from build123d import *

# Parameters (mm, degrees)
SKETCH1_W           = 457.2
SKETCH1_H           = 304.8
BOSS_EXTRUDE1_DEPTH = 3.175
CUT_EXTRUDE1_DEPTH  = 4.175
CUT_EXTRUDE2_REACH  = 5.175
SKETCH5_R           = 1.700000029
CUT_EXTRUDE3_DEPTH  = 4.175
SKETCH7_R           = 2.200000045
CUT_EXTRUDE5_DEPTH  = 4.175
SKETCH8_R           = 1.000000032
CUT_EXTRUDE6_DEPTH  = 4.175
SKETCH12_R          = 1.700000029
CUT_EXTRUDE7_DEPTH  = 4.175
SKETCH13_R          = 1.700000029
SKETCH13_R_2        = 1.127000032
CUT_EXTRUDE8_DEPTH  = 4.175
SKETCH14_R          = 2.200000045
SKETCH14_R_2        = 1.700000029
SKETCH14_R_3        = 2.499999953
CUT_EXTRUDE9_DEPTH  = 4.175


with BuildPart() as part:
    # Sketch1 → Boss-Extrude1 (new body)
    with BuildSketch(Plane(origin=(0, 0, 0), x_dir=(1, 0, 0), z_dir=(0, 1, 0))):
        Rectangle(SKETCH1_W, SKETCH1_H)
    extrude(amount=BOSS_EXTRUDE1_DEPTH)

    # Sketch2 → Cut-Extrude1 (cut, through all)
    with BuildSketch(Plane(origin=(0, 3.175, 0), x_dir=(1, 0, 0), z_dir=(0, 1, 0))):
        with BuildLine():
            Line((-218.100000045, 66.04), (-218.100000045, 66.675))
            ThreePointArc((-218.100000045, 66.675), (-215.9, 68.875000045), (-213.699999955, 66.675))
            Line((-213.699999955, 66.675), (-213.699999955, 66.04))
            ThreePointArc((-213.699999955, 66.04), (-215.9, 63.839999955), (-218.100000045, 66.04))
        make_face()
        with BuildLine():
            Line((-186.350000045, 66.04), (-186.350000045, 66.675))
            ThreePointArc((-186.350000045, 66.675), (-184.15, 68.875000045), (-181.949999955, 66.675))
            Line((-181.949999955, 66.675), (-181.949999955, 66.04))
            ThreePointArc((-181.949999955, 66.04), (-184.15, 63.839999955), (-186.350000045, 66.04))
        make_face()
        with BuildLine():
            Line((-213.699999955, -66.04), (-213.699999955, -66.675))
            ThreePointArc((-213.699999955, -66.675), (-215.9, -68.875000045), (-218.100000045, -66.675))
            Line((-218.100000045, -66.675), (-218.100000045, -66.04))
            ThreePointArc((-218.100000045, -66.04), (-215.9, -63.839999955), (-213.699999955, -66.04))
        make_face()
        with BuildLine():
            Line((-181.949999955, -66.04), (-181.949999955, -66.675))
            ThreePointArc((-181.949999955, -66.675), (-184.15, -68.875000045), (-186.350000045, -66.675))
            Line((-186.350000045, -66.675), (-186.350000045, -66.04))
            ThreePointArc((-186.350000045, -66.04), (-184.15, -63.839999955), (-181.949999955, -66.04))
        make_face()
    extrude(amount=-CUT_EXTRUDE1_DEPTH, mode=Mode.SUBTRACT)

    # Sketch4 → Cut-Extrude2 (cut, up to next)
    with BuildSketch(Plane(origin=(0, 3.175, 0), x_dir=(1, 0, 0), z_dir=(0, 1, 0)), mode=Mode.PRIVATE) as cut_extrude2_sk1:
        with BuildLine():
            Line((-185.7375, 46.0375), (-185.7375, -46.0375))
            Line((-185.7375, -46.0375), (-180.34, -46.0375))
            ThreePointArc((-180.34, -46.0375), (-179.666480791, -46.316480791), (-179.3875, -46.99))
            Line((-179.3875, -46.99), (-179.3875, -55.3085))
            Line((-179.3875, -55.3085), (-70.0405, -55.3085))
            Line((-70.0405, -55.3085), (-70.0405, 55.3085))
            Line((-70.0405, 55.3085), (-179.3875, 55.3085))
            Line((-179.3875, 55.3085), (-179.3875, 46.99))
            ThreePointArc((-179.3875, 46.99), (-179.666480791, 46.316480791), (-180.34, 46.0375))
            Line((-180.34, 46.0375), (-185.7375, 46.0375))
        make_face()
    cut_extrude2_tool1 = extrude(cut_extrude2_sk1.sketch, amount=-CUT_EXTRUDE2_REACH, mode=Mode.PRIVATE) & part.part
    add(cut_extrude2_tool1.solids().sort_by_distance((-127.382939, 3.175, 0))[0], mode=Mode.SUBTRACT)

    # Sketch5 → Cut-Extrude3 (cut, through all)
    with BuildSketch(Plane(origin=(0, 3.175, 0), x_dir=(1, 0, 0), z_dir=(0, 1, 0))):
        with Locations((-203.2, 79.629)):
            Circle(SKETCH5_R)
        with Locations((-222.25, 143.129)):
            Circle(SKETCH5_R)
        with Locations((-222.25, 79.629)):
            Circle(SKETCH5_R)
        with Locations((-203.2, -79.629)):
            Circle(SKETCH5_R)
        with Locations((-222.25, -79.629)):
            Circle(SKETCH5_R)
        with Locations((-222.25, -143.129)):
            Circle(SKETCH5_R)
    extrude(amount=-CUT_EXTRUDE3_DEPTH, mode=Mode.SUBTRACT)

    # Sketch7 → Cut-Extrude5 (cut, through all)
    with BuildSketch(Plane(origin=(0, 3.175, 0), x_dir=(1, 0, 0), z_dir=(0, 1, 0))):
        with Locations((-50.720000033, -132.250000041)):
            Circle(SKETCH7_R)
        with Locations((-40.719999967, -132.250000041)):
            Circle(SKETCH7_R)
        with Locations((-50.720000033, -83.649999959)):
            Circle(SKETCH7_R)
        with Locations((-40.719999967, -83.649999959)):
            Circle(SKETCH7_R)
        Polygon((-55.846999939, -87.373000006), (-46.22, -87.373000006), (-46.22, -80.769000006), (-45.22, -80.769000006), (-45.22, -87.373000006), (-35.593000061, -87.373000006), (-35.593000061, -128.526999994), (-45.22, -128.526999994), (-45.22, -135.130999994), (-46.22, -135.130999994), (-46.22, -128.526999994), (-55.846999939, -128.526999994), align=None)
    cut_extrude5 = extrude(amount=-CUT_EXTRUDE5_DEPTH, mode=Mode.SUBTRACT)

    # Mirror1: Cut-Extrude5 across plane
    add(cut_extrude5.mirror(Plane.XY), mode=Mode.SUBTRACT)

    # Sketch8 → Cut-Extrude6 (cut, through all)
    with BuildSketch(Plane(origin=(0, 3.175, 0), x_dir=(1, 0, 0), z_dir=(0, 1, 0))):
        with Locations((-63.6905, -38.1)):
            Circle(SKETCH8_R)
        with Locations((-63.6905, -12.7)):
            Circle(SKETCH8_R)
        with Locations((-63.6905, 12.7)):
            Circle(SKETCH8_R)
        with Locations((-63.6905, 38.1)):
            Circle(SKETCH8_R)
    extrude(amount=-CUT_EXTRUDE6_DEPTH, mode=Mode.SUBTRACT)

    # Sketch12 → Cut-Extrude7 (cut, through all)
    with BuildSketch(Plane(origin=(0, 3.175, 0), x_dir=(1, 0, 0), z_dir=(0, 1, 0))):
        with Locations((195.024, -95.25)):
            Circle(SKETCH12_R)
        with Locations((182.324, -95.25)):
            Circle(SKETCH12_R)
        with Locations((195.024, -146.05)):
            Circle(SKETCH12_R)
        with Locations((182.324, -146.05)):
            Circle(SKETCH12_R)
        with Locations((167.9575, -95.25)):
            Circle(SKETCH12_R)
        with Locations((158.4325, -95.25)):
            Circle(SKETCH12_R)
        with Locations((167.9575, -146.05)):
            Circle(SKETCH12_R)
        with Locations((158.4325, -146.05)):
            Circle(SKETCH12_R)
        with Locations((21.9075, -146.05)):
            Circle(SKETCH12_R)
        with Locations((12.3825, -146.05)):
            Circle(SKETCH12_R)
        with Locations((12.3825, -95.25)):
            Circle(SKETCH12_R)
        with Locations((21.9075, -95.25)):
            Circle(SKETCH12_R)
    extrude(amount=-CUT_EXTRUDE7_DEPTH, mode=Mode.SUBTRACT)

    # Sketch13 → Cut-Extrude8 (cut, through all)
    with BuildSketch(Plane(origin=(0, 3.175, 0), x_dir=(1, 0, 0), z_dir=(0, 1, 0))):
        with Locations((212.725, 95.25)):
            Circle(SKETCH13_R)
        with Locations((212.725, 146.05)):
            Circle(SKETCH13_R)
        with Locations((200.025, 95.25)):
            Circle(SKETCH13_R)
        with Locations((200.025, 146.05)):
            Circle(SKETCH13_R)
        with Locations((177.213, 133.477000026)):
            Circle(SKETCH13_R_2)
        with Locations((164.513, 143.002000026)):
            Circle(SKETCH13_R_2)
        with Locations((164.513, 123.952000026)):
            Circle(SKETCH13_R_2)
        with Locations((34.925, 95.25)):
            Circle(SKETCH13_R)
        with Locations((34.925, 146.05)):
            Circle(SKETCH13_R)
        with Locations((22.225, 95.25)):
            Circle(SKETCH13_R)
        with Locations((22.225, 146.05)):
            Circle(SKETCH13_R)
        with Locations((-0.587, 133.477000026)):
            Circle(SKETCH13_R_2)
        with Locations((-13.287, 143.002000026)):
            Circle(SKETCH13_R_2)
        with Locations((-13.287, 123.952000026)):
            Circle(SKETCH13_R_2)
    extrude(amount=-CUT_EXTRUDE8_DEPTH, mode=Mode.SUBTRACT)

    # Sketch14 → Cut-Extrude9 (cut, through all)
    with BuildSketch(Plane(origin=(0, 3.175, 0), x_dir=(1, 0, 0), z_dir=(0, 1, 0))):
        with Locations((49.758847455, 40.411152545)):
            Circle(SKETCH14_R)
        with Locations((130.581152545, 40.411152545)):
            Circle(SKETCH14_R)
        with Locations((49.758847455, -40.411152545)):
            Circle(SKETCH14_R)
        with Locations((130.581152545, -40.411152545)):
            Circle(SKETCH14_R)
        with Locations((-20.833999988, 15.499999988)):
            Circle(SKETCH14_R_2)
        with Locations((10.165999988, 15.499999988)):
            Circle(SKETCH14_R_2)
        with Locations((-20.833999988, -15.499999988)):
            Circle(SKETCH14_R_2)
        with Locations((10.165999988, -15.499999988)):
            Circle(SKETCH14_R_2)
        with Locations((-5.334, 0)):
            Circle(SKETCH14_R_3)
    extrude(amount=-CUT_EXTRUDE9_DEPTH, mode=Mode.SUBTRACT)


solid = part.part
Check sheet for the modelled part. Datum: model origin and axes. Units: mm. Give positions to 0.01 mm unless a question says otherwise; leave off trailing zeros. Write each loop counter-clockwise with the first axis right and the second up, starting at its lowest first coordinate (ties: lowest second). Pieces come first, ordered by that corner, then holes. Notation, with made-up numbers: M 50,-20 L 102,-20 A36 ccw 102,16 Z; hole C 5,32 d5. An arc over 180 degrees is marked long. Use one line per item in the form item = value.
(1) Material ranges on line 1 along Z through (x, y) = (22.5, 0.2); line 2 along Z through (x, y) = (-203.2, 1.2); line 3 along Z through (x, y) = (194.5, 3.05), recorded low to high.
Answer block:
line_1 = -152.4 to -147.73, -144.37 to -96.93, -93.57 to 93.66, 96.84 to 144.46, 147.64 to 152.4
line_2 = -152.4 to -81.33, -77.93 to 77.93, 81.33 to 152.4
line_3 = -152.4 to 93.63, 96.87 to 144.43, 147.67 to 152.4
(2) Section check C-C on y = 2.1. State how many separate pieces and enclosed holes the cut face has, plus the area to 3 significant figures.
Answer block:
separate_pieces = 1
enclosed_holes = 60
area = 124,000 mm2
(3) Section check B-B on z = 27. Record the boundary of the cut face in (x, y) (1 decimal), plus the area to 3 significant figures.
Answer block:
outline = M -228.6,0 L -185.7,0 L -185.7,3.2 L -228.6,3.2 Z; M -70,0 L 228.6,0 L 228.6,3.2 L -70,3.2 Z
area = 1,080 mm2
(4) Section check A-A on x = -139. Record the boundary of the cut face in (y, z) (1 decimal).
Answer block:
outline = M 0,-152.4 L 3.2,-152.4 L 3.2,-55.3 L 0,-55.3 Z; M 0,55.3 L 3.2,55.3 L 3.2,152.4 L 0,152.4 Z
(5) Depth check by flat-ended pin: P1, Ø3, axis at x = 158.43, z = 146.05, coming from the -Y side. Enter the tip coordinate at first touch or a pass-through.
Answer block:
P1 = through
